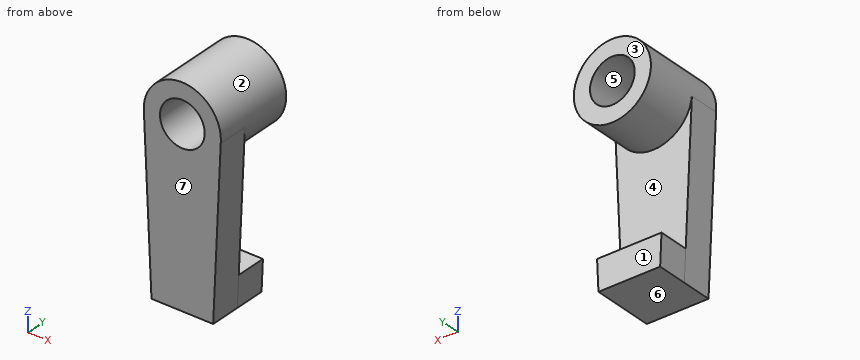
from build123d import *

# Parameters (mm, degrees)
F0_R     = 15.875
F0_R_2   = 9.2075
F1_DEPTH = 34.29
F3_DEPTH = 12.7
F5_DEPTH = 12.7


with BuildPart() as f1:
    # F0 (on Front) → F1 (new body)
    with BuildSketch(Plane.XZ):
        Circle(F0_R)
        Circle(F0_R_2, mode=Mode.SUBTRACT)
    extrude(amount=F1_DEPTH)

    # F2 (on face) → F3 (join)
    with BuildSketch(Plane.XZ.offset(34.29)):
        with BuildLine():
            ThreePointArc((15.8118485958, -1.4145914552), (15.8592042905, -0.7080001915), (15.875, 0))
            Line((15.875, 0), (15.8118485958, -1.4145914552))
        make_face()
        with BuildLine():
            ThreePointArc((-15.875, 0), (-15.8592042905, -0.7080001915), (-15.8118485958, -1.4145914552))
            Line((-15.8118485958, -1.4145914552), (-15.875, 0))
        make_face()
        with BuildLine():
            Line((12.7, -71.12), (15.8118485958, -1.4145914552))
            ThreePointArc((15.8118485958, -1.4145914552), (0, -15.875), (-15.8118485958, -1.4145914552))
            Line((-15.8118485958, -1.4145914552), (-12.7, -71.12))
            Line((-12.7, -71.12), (12.7, -71.12))
        make_face()
    extrude(amount=-F3_DEPTH)

    # F4 (on face) → F5 (join)
    with BuildSketch(Plane(origin=(0, -21.59, 0), x_dir=(-1, 0, 0), z_dir=(0, 1, 0))):
        Polygon((-13.2669642857, -58.42), (-12.7, -71.12), (12.7, -71.12), (13.2669642857, -58.42), align=None)
    extrude(amount=F5_DEPTH)


solid = f1.part
Geometry check sheet. Reference: the model listing, model coordinates, mm. Face numbers are marked on the shaded views. A direction names the side the tool comes from. Coordinates: 2 decimals unless noted, no trailing zeros. Order: outer loops, then holes, each group sorted by start corner. A loop starts at its lowest first (then second) coordinate and runs counter-clockwise, first axis right, second up. Notation, with made-up numbers: (20, 48) -> (71, 48) arc R6 ccw to (71, 59) -> close; hole circle Ø8 at (-16.5, 35). An arc over 180 degrees is marked (long way). Use a Markdown table: item, result. Add a question column.
1. Cross-section at B-B (y = -19). Give the number of separate pieces and of enclosed holes in the cut face, and give its area (3 significant figures).
2. Material ranges on L1, parallel to Z at x = 0, y = -10 (1 decimal); L2, parallel to Z at x = 2, y = -14; L3, parallel to Z at x = 0, y = -27 (1 decimal), recorded low to high.
3. Set-up check for the marked faces 1, 2 and 3: record each of +Z, -Z, +X, -X, +Y, -Y from which the full face is reachable in a straight line by a thin tool's end or side.
4. Cross-section at C-C (z = 0). Enter the section's corners in (x, y) (1 decimal).
5. Mould release check, pull along Z, two halves, no side actions. Record for the marked faces 4, 5, 6 and 7: pulls with the +Z half, pulls with the -Z half, needs draft (parallel to the pull), parting line crosses it, or undercut.
6. Cross-section at A-A (x = 0). Enter the section's corners in (y, z) (1 decimal), and give its area (3 significant figures).
7. Go/stop test with flat-tipped pins: pin 1 Ø5 at (x, y) = (-6, -10.5) entering from +Z; pin 2 Ø10 at (y, z) = (-23, -9) entering from +X; pin 3 Ø4 at (y, z) = (-5.5, -13.5) entering from -X. Record where each tip stops, or that it passes through.
Filled sheet:
| question | item | result |
|---|---|---|
| 1 | separate pieces | 2 |
| 1 | enclosed holes | 1 |
| 1 | area | 855 mm2 |
| 2 | L1 | -71.1 to -58.4, -15.9 to -9.2, 9.2 to 15.9 |
| 2 | L2 | -71.12 to -58.42, -15.75 to -8.99, 8.99 to 15.75 |
| 2 | L3 | -71.1 to -9.2, 9.2 to 15.9 |
| 3 | face 1 | -Z, +X, -X, +Y |
| 3 | face 2 | +Y |
| 3 | face 3 | +Z, -Z, +X, -X, +Y |
| 4 | outline | (-15.9, -34.3) -> (-9.2, -34.3) -> (-9.2, 0) -> (-15.9, 0) -> close; (9.2, -34.3) -> (15.9, -34.3) -> (15.9, 0) -> (9.2, 0) -> close |
| 5 | face 4 | undercut |
| 5 | face 5 | undercut |
| 5 | face 6 | pulls with the -Z half |
| 5 | face 7 | needs draft |
| 6 | outline | (-34.3, -71.1) -> (-8.9, -71.1) -> (-8.9, -58.4) -> (-21.6, -58.4) -> (-21.6, -15.9) -> (0, -15.9) -> (0, -9.2) -> (-34.3, -9.2) -> close; (-34.3, 9.2) -> (0, 9.2) -> (0, 15.9) -> (-34.3, 15.9) -> close |
| 6 | area | 1,320 mm2 |
| 7 | pin 1 | z = 15.48 |
| 7 | pin 2 | x = 15.7 |
| 7 | pin 3 | x = -10.94 |
